from build123d import *

# Parameters (mm, degrees)
SKETCH1_W           = 270
SKETCH1_H           = 200
BOSS_EXTRUDE1_DEPTH = 10
SKETCH10_W          = 40
SKETCH10_H          = 50
CUT_EXTRUDE1_DEPTH  = 5
SKETCH10_3_W        = 40
SKETCH10_3_H        = 50
BOSS_EXTRUDE2_DEPTH = 5
SKETCH12_R          = 3
CUT_EXTRUDE2_DEPTH  = 5
SKETCH12_3_R        = 3
CUT_EXTRUDE3_DEPTH  = 5
BOSS_EXTRUDE3_DEPTH = 50
CUT_EXTRUDE4_REACH  = 341.706
SKETCH15_R          = 2.75
CUT_EXTRUDE5_REACH  = 341.706
SKETCH16_R          = 3
SKETCH17_W          = 230
SKETCH17_H          = 10
CUT_EXTRUDE6_DEPTH  = 15
CUT_EXTRUDE7_REACH  = 341.006
SKETCH18_W          = 240
SKETCH18_H          = 200
BOSS_EXTRUDE4_DEPTH = 10
FILLET1_R           = 3


with BuildPart() as part:
    # Sketch1 → Boss-Extrude1 (new body)
    with BuildSketch(Plane(origin=(0, 0, 0), x_dir=(1, 0, 0), z_dir=(0, 1, 0))):
        with Locations((135, 100)):
            Rectangle(SKETCH1_W, SKETCH1_H)
    extrude(amount=-BOSS_EXTRUDE1_DEPTH)

    # Sketch10 → Cut-Extrude1 (cut)
    with BuildSketch(Plane(origin=(0, 0, 0), x_dir=(1, 0, 0), z_dir=(0, 1, 0))):
        with Locations((20, 150)):
            Rectangle(SKETCH10_W, SKETCH10_H)
    extrude(amount=-CUT_EXTRUDE1_DEPTH, mode=Mode.SUBTRACT)

    # Sketch10_3 → Boss-Extrude2 (add)
    with BuildSketch(Plane(origin=(0, 0, 0), x_dir=(1, 0, 0), z_dir=(0, 1, 0))):
        with Locations((-20, 50)):
            Rectangle(SKETCH10_3_W, SKETCH10_3_H)
    extrude(amount=-BOSS_EXTRUDE2_DEPTH)

    # Sketch12 → Cut-Extrude2 (cut)
    with BuildSketch(Plane(origin=(0, -5, 0), x_dir=(1, 0, 0), z_dir=(0, 1, 0))):
        with Locations(Location((25, 150, 0), (0, 0, 270))):
            Circle(SKETCH12_R)
    extrude(amount=-CUT_EXTRUDE2_DEPTH, mode=Mode.SUBTRACT)

    # Sketch12_3 → Cut-Extrude3 (cut)
    with BuildSketch(Plane(origin=(0, -5, 0), x_dir=(1, 0, 0), z_dir=(0, 1, 0))):
        with Locations(Location((-25, 50, 0), (0, 0, 270))):
            Circle(SKETCH12_3_R)
    extrude(amount=CUT_EXTRUDE3_DEPTH, mode=Mode.SUBTRACT)

    # Sketch13 → Boss-Extrude3 (add)
    with BuildSketch(Plane(origin=(0, 0, 0), x_dir=(1, 0, 0), z_dir=(0, 1, 0))):
        Polygon((0, 190), (260, 190), (260, 10), (0, 10), (0, 0), (270, 0), (270, 200), (0, 200), align=None)
    extrude(amount=BOSS_EXTRUDE3_DEPTH)

    # Sketch15 → Cut-Extrude4 (cut, up to next)
    with BuildSketch(Plane(origin=(0, 0, 0), x_dir=(1, 0, 0), z_dir=(0, 1, 0)), mode=Mode.PRIVATE) as cut_extrude4_sk1:
        with Locations(Location((230, 78.5, 0), (0, 0, 270))):
            Circle(SKETCH15_R)
    cut_extrude4_tool1 = extrude(cut_extrude4_sk1.sketch, amount=-CUT_EXTRUDE4_REACH, mode=Mode.PRIVATE) & part.part
    # Sketch15 → Cut-Extrude4 (cut, up to next)
    with BuildSketch(Plane(origin=(0, 0, 0), x_dir=(1, 0, 0), z_dir=(0, 1, 0)), mode=Mode.PRIVATE) as cut_extrude4_sk2:
        with Locations(Location((230, 121.5, 0), (0, 0, 270))):
            Circle(SKETCH15_R)
    cut_extrude4_tool2 = extrude(cut_extrude4_sk2.sketch, amount=-CUT_EXTRUDE4_REACH, mode=Mode.PRIVATE) & part.part
    add(cut_extrude4_tool1.solids().sort_by_distance((230, 0, -78.5))[0], mode=Mode.SUBTRACT)
    add(cut_extrude4_tool2.solids().sort_by_distance((230, 0, -121.5))[0], mode=Mode.SUBTRACT)

    # Sketch16 → Cut-Extrude5 (cut, up to next)
    with BuildSketch(Plane(origin=(0, 0, 0), x_dir=(1, 0, 0), z_dir=(0, 1, 0)), mode=Mode.PRIVATE) as cut_extrude5_sk1:
        with Locations(Location((230, 143, 0), (0, 0, 270))):
            Circle(SKETCH16_R)
    cut_extrude5_tool1 = extrude(cut_extrude5_sk1.sketch, amount=-CUT_EXTRUDE5_REACH, mode=Mode.PRIVATE) & part.part
    # Sketch16 → Cut-Extrude5 (cut, up to next)
    with BuildSketch(Plane(origin=(0, 0, 0), x_dir=(1, 0, 0), z_dir=(0, 1, 0)), mode=Mode.PRIVATE) as cut_extrude5_sk2:
        with Locations(Location((230, 175, 0), (0, 0, 270))):
            Circle(SKETCH16_R)
    cut_extrude5_tool2 = extrude(cut_extrude5_sk2.sketch, amount=-CUT_EXTRUDE5_REACH, mode=Mode.PRIVATE) & part.part
    # Sketch16 → Cut-Extrude5 (cut, up to next)
    with BuildSketch(Plane(origin=(0, 0, 0), x_dir=(1, 0, 0), z_dir=(0, 1, 0)), mode=Mode.PRIVATE) as cut_extrude5_sk3:
        with Locations(Location((230, 57, 0), (0, 0, 270))):
            Circle(SKETCH16_R)
    cut_extrude5_tool3 = extrude(cut_extrude5_sk3.sketch, amount=-CUT_EXTRUDE5_REACH, mode=Mode.PRIVATE) & part.part
    # Sketch16 → Cut-Extrude5 (cut, up to next)
    with BuildSketch(Plane(origin=(0, 0, 0), x_dir=(1, 0, 0), z_dir=(0, 1, 0)), mode=Mode.PRIVATE) as cut_extrude5_sk4:
        with Locations(Location((230, 25, 0), (0, 0, 270))):
            Circle(SKETCH16_R)
    cut_extrude5_tool4 = extrude(cut_extrude5_sk4.sketch, amount=-CUT_EXTRUDE5_REACH, mode=Mode.PRIVATE) & part.part
    add(cut_extrude5_tool1.solids().sort_by_distance((230, 0, -143))[0], mode=Mode.SUBTRACT)
    add(cut_extrude5_tool2.solids().sort_by_distance((230, 0, -175))[0], mode=Mode.SUBTRACT)
    add(cut_extrude5_tool3.solids().sort_by_distance((230, 0, -57))[0], mode=Mode.SUBTRACT)
    add(cut_extrude5_tool4.solids().sort_by_distance((230, 0, -25))[0], mode=Mode.SUBTRACT)

    # Sketch17 → Cut-Extrude6 (cut)
    with BuildSketch(Plane(origin=(0, 50, 0), x_dir=(1, 0, 0), z_dir=(0, 1, 0))):
        with Locations((115, 5)):
            Rectangle(SKETCH17_W, SKETCH17_H)
        with Locations((115, 195)):
            Rectangle(SKETCH17_W, SKETCH17_H)
    extrude(amount=-CUT_EXTRUDE6_DEPTH, mode=Mode.SUBTRACT)

    # Sketch18 → Cut-Extrude7 (cut, up to next)
    with BuildSketch(Plane(origin=(0, 35, 0), x_dir=(1, 0, 0), z_dir=(0, 1, 0)), mode=Mode.PRIVATE) as cut_extrude7_sk1:
        with Locations((80, 100)):
            Rectangle(SKETCH18_W, SKETCH18_H)
    cut_extrude7_tool1 = extrude(cut_extrude7_sk1.sketch, amount=-CUT_EXTRUDE7_REACH, mode=Mode.PRIVATE) & part.part
    add(cut_extrude7_tool1.solids().sort_by_distance((80, 35, -100))[0], mode=Mode.SUBTRACT)

    # Sketch14 → Boss-Extrude4 (add)
    with BuildSketch(Plane.XZ.offset(10)):
        Polygon((200, -190), (260, -190), (260, -160), (270, -160), (270, -200), (200, -200), align=None)
        Polygon((270, 0), (200, 0), (200, -10), (260, -10), (260, -40), (270, -40), align=None)
    extrude(amount=BOSS_EXTRUDE4_DEPTH)

    # Fillet1
    fillet1_edges = [part.edges().sort_by_distance(p)[0] for p in [
        (230, 42.5, 0),
        (230, 42.5, -10),
        (230, 42.5, -190),
        (230, 42.5, -200),
        (200, 17.5, -190),
        (200, 17.5, -10),
        (200, 7.5, 0),
        (200, 7.5, -200),
        (200, -15, -190),
        (270, -15, -160),
        (260, -15, -160),
        (260, -15, -190),
        (260, -15, -10),
        (260, -15, -40),
        (270, -15, -40),
        (200, -15, -10),
        (260, 25, -190),
        (260, 25, -10),
        (270, 15, 0),
        (270, 15, -200),
    ]]
    fillet(fillet1_edges, radius=FILLET1_R)


solid = part.part
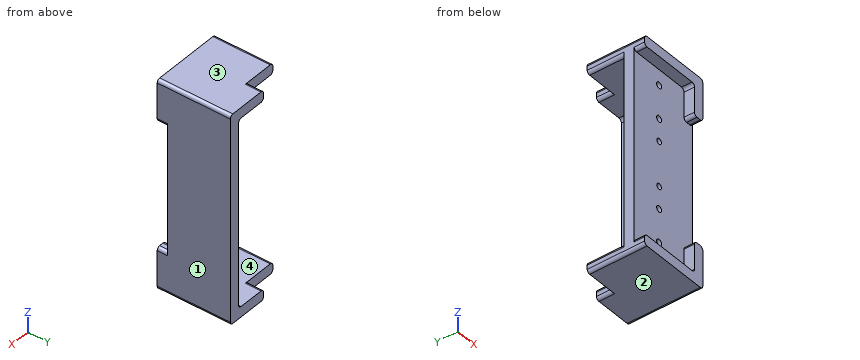
Input: part model. Units: mm. Frame: model coordinates. Face numbers are marked on the shaded views. Give positions to 0.01 mm unless a question says otherwise; leave off trailing zeros. Order: outer loops, then holes, each group sorted by start corner. A loop starts at its lowest first (then second) coordinate and runs counter-clockwise, first axis right, second up.
Q1. Contact query for flat-ended pins moving along their axis: pin 1 Ø3.5 at (x, z) = (230, -25) entering from -Y; pin 2 Ø3 at (x, z) = (217.5, -7) entering from +Y; pin 3 Ø1 at (x, z) = (222.5, -161.5) entering from +Y; pin 4 Ø15 at (y, z) = (13, -91.5) entering from -X. Output: stop coordinate, or through.
Checked values:
pin 1: passes through
pin 2: stops at y = 35
pin 3: stops at y = 0
pin 4: stops at x = 260
Q2. Section D-D on z = -175. Output: boundary loops of the cut face in (x, y).
Checked values:
outline: (200, -10) - (227, -10) - (227, 0) - (200, 0) - close; (233, -10) - (260, -10) - (260, -20) - (270, -20) - (270, 50) - (260, 50) - (260, 0) - (233, 0) - close
Q3. Draft query along Z for the marked faces 1, 2, 3 and 4. Return one class per face: +Z half, -Z half, draft (parallel to the pull), parting line (faces both ways), or undercut.
Checked values:
face 1: draft
face 2: -Z half
face 3: +Z half
face 4: undercut
Q4. Section A-A on z = -121.5. Output: boundary loops of the cut face in (x, y), and give its area (4 significant figures).
Checked values:
outline: (200, -10) - (227.25, -10) - (227.25, 0) - (200, 0) - close; (232.75, -10) - (270, -10) - (270, 50) - (260, 50) - (260, 0) - (232.75, 0) - close
area: 1,145 mm2
Q5. Section C-C on x = 254.5. Output: boundary loops of the cut face in (y, z).
Checked values:
outline: (-20, -200) - (50, -200) - (50, -190) - (0, -190) - (0, -10) - (50, -10) - (50, 0) - (-20, 0) - (-20, -10) - (-10, -10) - (-10, -190) - (-20, -190) - close
Q6. Ray query, probe 1 along Z at (x, y) = (241, 33); probe 2 along X at (y, z) = (-3.5, -25); probe 3 along Y at (x, z) = (229, -152.5). Return the intervals inside material, ascending.
Checked values:
probe 1: z = -200 to -190, -10 to 0
probe 2: x = 200 to 227, 233 to 270
probe 3: y = -10 to 0
Q7. Section B-B on y = -13. Output: boundary loops of the cut face in (x, z), and give its area (3 significant figures).
Checked values:
outline: (200, -197) arc R3 ccw to (203, -200) - (267, -200) arc R3 ccw to (270, -197) - (270, -163) arc R3 ccw to (267, -160) - (263, -160) arc R3 ccw to (260, -163) - (260, -187) arc R3 cw to (257, -190) - (203, -190) arc R3 ccw to (200, -193) - close; (200, -7) arc R3 ccw to (203, -10) - (257, -10) arc R3 cw to (260, -13) - (260, -37) arc R3 ccw to (263, -40) - (267, -40) arc R3 ccw to (270, -37) - (270, -3) arc R3 ccw to (267, 0) - (203, 0) arc R3 ccw to (200, -3) - close
area: 1,980 mm2
